The listing builds one solid part. Answer for the finished solid, in the listing's coordinates (mm). Round coordinates to 2 decimals unless told otherwise and drop trailing zeros. Write each loop counter-clockwise with the first axis right and the second up, starting at its lowest first coordinate (ties: lowest second). Pieces come first, ordered by that corner, then holes. Notation, with made-up numbers: M 71,37 L 116,37 A17 ccw 116,53 Z; hole C -35.5,52 d1. An arc over 180 degrees is marked long. Answer as CSV lines item,"result". Start each with the question number.
Autodesk Inventor part; units mm, degrees
ref_plane "YZ Plane" through (0, 0, 0) normal (1, 0, 0) x (0, 1, 0)
ref_plane "XZ Plane" through (0, 0, 0) normal (0, 1, 0) x (-1, 0, 0)
ref_plane "XY Plane" through (0, 0, 0) normal (0, 0, 1) x (1, 0, 0)
sketch "Sketch1" plane through (0, 0, 0) normal (0, 0, 1) x (1, 0, 0)
  line L0 (-17.78, 0) -> (17.78, 0)
  line L1 (0, -17.78) -> (0, 17.78)
  line L2 (-12.7, 12.7) -> (12.7, 12.7)
  line L3 (12.7, 12.7) -> (12.7, -12.7)
  line L4 (12.7, -12.7) -> (-12.7, -12.7)
  line L5 (-12.7, -12.7) -> (-12.7, 12.7)
  line L6 (9.525, 9.525) -> (-9.525, 9.525)
  line L7 (-9.525, 9.525) -> (-9.525, -9.525)
  line L8 (-9.525, -9.525) -> (9.525, -9.525)
  line L9 (9.525, -9.525) -> (9.525, 9.525)
  point P0 (0, 0)
  point P1 (-12.7, 0)
  point P2 (0, 12.7)
  dimension "d0" = 25.4
  dimension "d1" = 3.175
extrude "Extrusion1" add sketch "Sketch1" along normal mid plane 254 contours L5 L2 L1 L6 L7 L0 | L0 L7 L8 L1 L4 L5 | L1 L8 L9 L0 L3 L4 | L2 L3 L0 L9 L6 L1
sketch "Sketch3" plane through (-12.7, 12.7, 127) normal (0, 1, 0) x (1, 0, 0)
  line L0 (25.4, 0) -> (25.4, 254)
  line L1 (25.4, 254) -> (0, 254)
  line L2 (0, 254) -> (25.4, 234.5099)
  point P0 (12.7, 127)
  dimension "d7" = 37.5
extrude "Extrusion3" cut sketch "Sketch3" against normal through all
sketch "Sketch4" plane through (-12.7, 12.7, 127) normal (0, 1, 0) x (1, 0, 0)
  line L0 (0, 0) -> (25.4, 0)
  line L1 (25.4, 0) -> (25.4, 234.5099)
  line L2 (0, 0) -> (25.4, 6.8059)
  point P0 (12.7, 127)
  dimension "d10" = 15
extrude "Extrusion4" cut sketch "Sketch4" against normal through all
properties part number "tubing_template_0.125" material "Aluminum-6061"
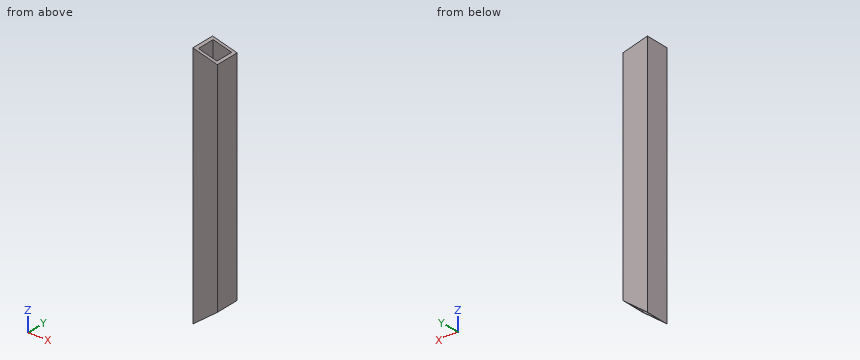
Q1. Straight lines are drawn through the part: L1, parallel to Y at x = 2, z = 74.5 (3 decimals); L2, parallel to Z at x = -2.25, y = -11.5. For each, find the intervals that lie inside material, in ascending order.
Q2. Find section A-A (z = 21). Determine the outline of the cut face in (x, y) (3 decimals), plus the area to 3 significant figures.
Q3. Find section B-B (y = -2.75). Determine the outline of the cut face in (x, z) (3 decimals), plus the area to 3 significant figures.
Q4. Each of these flat-tipped pins is pushed along its axis until it touches: P1, Ø10, axis at x = -7, y = 5, coming from the -Z side; P2, Ø12, axis at x = -5.5, y = 3.5, coming from the +Z side; P3, Ø2, axis at x = 9.5, y = 8, coming from the -Z side. Where does it stop, or does it pass through?
Q5. Find section C-C (x = -5.5). Determine the outline of the cut face in (y, z) (3 decimals), plus the area to 3 significant figures.
Reported:
1,L1,"y = -12.7 to -9.525, 9.525 to 12.7"
1,L2,"z = -118.98 to 124.2"
2,outline,"M -12.7,-12.7 L 12.7,-12.7 L 12.7,12.7 L -12.7,12.7 Z; hole M -9.525,-9.525 L 9.525,-9.525 L 9.525,9.525 L -9.525,9.525 Z"
2,area,"282 mm2"
3,outline,"M -12.7,-127 L -9.525,-124.564 L -9.525,126.149 L -12.7,127 Z; M 9.525,-109.946 L 12.7,-107.51 L 12.7,120.194 L 9.525,121.045 Z"
3,area,"1,530 mm2"
4,P1,"stops at z = -126.46"
4,P2,"stops at z = 126.68"
4,P3,"stops at z = -109.95"
5,outline,"M -12.7,-121.475 L -9.525,-121.475 L -9.525,125.071 L -12.7,125.071 Z; M 9.525,-121.475 L 12.7,-121.475 L 12.7,125.071 L 9.525,125.071 Z"
5,area,"1,570 mm2"
